Part model, mm, in its own coordinate system. Round coordinates to 2 decimals unless told otherwise and drop trailing zeros. Use CSV: the item, a comma, the result in double quotes. Start each with the question number.
Solid Edge part; units mm, degrees
sketch "Sketch1" plane through (0, 0, 0) normal (0, 0, 1) x (1, 0, 0)
  circle A0 centre (0, 0) radius 28
extrude "Protrusion1" add sketch "Sketch1" along normal blind 2
sketch "Sketch2" plane through (0, 0, 0) normal (0, 0, -1) x (0, -1, 0)
  circle A0 centre (0, 0) radius 23
extrude "ExtrudedProtrusion_2" add sketch "Sketch2" along normal blind 1
sketch "Sketch3" plane through (0, 0, 0) normal (0, 0, 1) x (1, 0, 0)
  circle A0 centre (0, 14) radius 2.7
extrude "Cutout1" cut sketch "Sketch3" along normal through all and the other way through all
pattern_circular "Pattern1" count 3 over 360 about axis through (0, 0, 2) along (0, 0, -1) of "Cutout1"
sketch "Sketch4" plane through (0, 0, 0) normal (0, 0, 1) x (1, 0, 0)
  circle A0 centre (0, 0) radius 4.1
extrude "Cutout4" cut sketch "Sketch4" along normal through all and the other way through all
sketch "Sketch5" plane through (0, 0, -1) normal (0, 0, -1) x (0, 1, 0)
  line L0 (0, 9.798) -> (0, 16.8819)
  arc A0 (2.2353, 18.8681) -> (0, 16.8819) centre (2, 16.8819) ccw
  arc A1 (14.8383, 8.0513) -> (15.518, 10.9632) centre (13.8845, 9.8092) ccw
  line L1 (8.6119, 4.6728) -> (14.8383, 8.0513)
  arc A2 (6.1264, 5.1446) -> (8.6119, 4.6728) centre (7.6581, 6.4307) ccw
  arc A3 (0, 9.798) -> (1.6, 7.8384) centre (2, 9.798) ccw
  arc A4 (6.1264, 5.1446) -> (1.6, 7.8384) centre (0, 0) ccw
  arc A5 (2.2353, 18.8681) -> (15.518, 10.9632) centre (0, 0) cw
extrude "Cutout5" cut sketch "Sketch5" along normal through all and the other way through all
pattern_circular "Pattern2" count 3 over 360 about axis through (0, 0, -1) along (0, 0, 1) of "Cutout5"
fillet "Round_1" radius 1 1 edges at (23, 0, 0)
chamfer "Chamfer_1" distance 1 angle 45 1 edges at (-28, 0, 0)
fillet "Round_2" radius 2 1 edges at (27, 0, 0)
properties material "ABS Plastic, medium impact"
1. Pull direction Y, two halves, no side cores. Call faces 1 (the cylindrical face through (4.094, -7.516, 0.521)), 2 (the flat face through (12, -21, 0)): released by +Y, released by -Y, zero draft, split by the parting line, or undercut.
2. Drill centre lines: line 1 along Y through (x, z) = (0, 1); line 2 along Y through (x, z) = (13.5, 1.4); line 3 along Y through (x, z) = (-7, 0.35). Where is each one in solid material? Low to high. Write a range as [from, to].
3. Band-saw the part on A-A (x = 0). Give the number of separate pieces and of enclosed holes in the cut face, then the cut area to 3 significant figures.
4. Flat gauge pin, fed straight in: pin 1 (1.5 mm diameter, centred on y = -2, z = 1, fed in from +X). Where does the tip first touch, or does it go through?
Answers below:
1,face 1,"undercut"
1,face 2,"zero draft"
2,line 1,"y = [-28, -19], [-8, -4.1], [4.1, 11.3], [16.7, 28]"
2,line 2,"y = [-24.53, -9.32], [-4.68, 0], [13.37, 24.53]"
2,line 3,"y = [-26.39, -17.66], [-12.12, 3.87], [12.12, 26.39]"
3,separate pieces,"4"
3,enclosed holes,"0"
3,area,"83.5 mm^2"
4,pin 1,"stops at x = 27.97"
